Design review of the part shown in the three views and the two pictorial views. Dimensions are in mm from the part's minimum x, y and z. Coordinates: 2 decimals unless noted, no trailing zeros. Loops run counter-clockwise (first coordinate to the right, second up) from the corner with the lowest first, then second, coordinate; pieces in that order, holes last. Notation, with made-up numbers: M 42,-14.75 L 69,-14.75 A24 ccw 69,7.25 Z; hole C 75,-35 d5. An arc over 180 degrees is marked long. Answer as a JSON object with one key per item and string values. Group by question number.
Item 1: Wall thickness on L1, parallel to Y at x = 50, z = 1.3: over which ranges is the line inside the solid? List them lowest first. Write a range as from..to.
Item 2: Add section B-B (x = 10). State the section outline as (y, z) points, then the cut area to 3 significant figures.
Item 3: Insertion check: pin 1 (1 mm diameter, centred on x = 15, z = 2.5, fed in from -Y). The pin has a flat end and moves straight along its axis. Give the tip position at first contact, or say it passes through.
Item 4: Add section A-A (y = 10). State the section outline as (x, z) points.
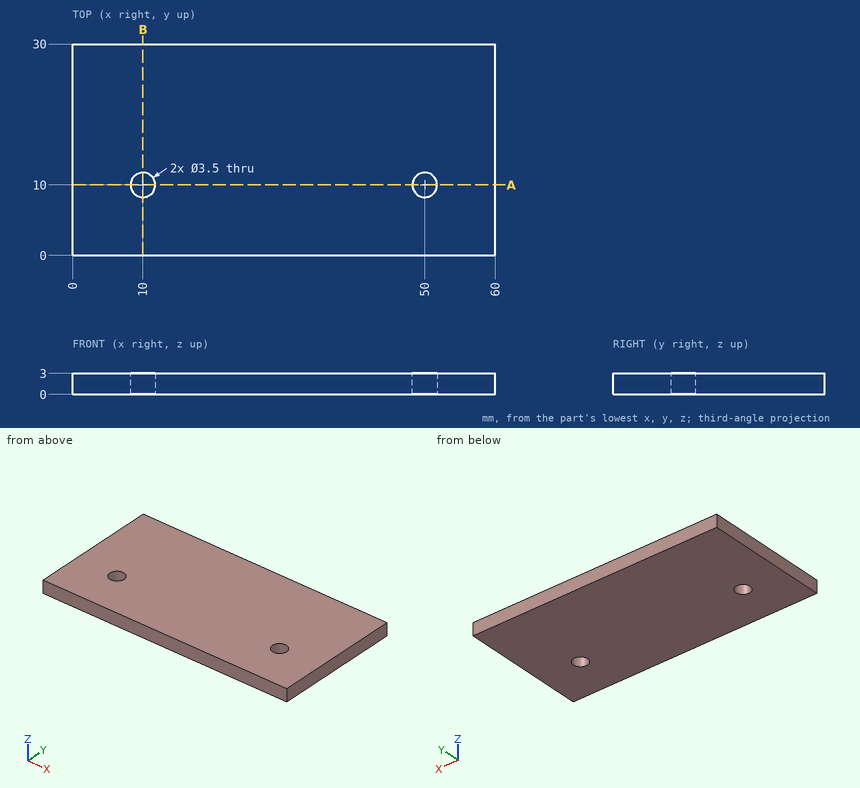
From the geometry:
{
 "1": {"L1": "y = 0..8.25, 11.75..30"},
 "2": {"outline": "M 0,0 L 8.25,0 L 8.25,3 L 0,3 Z; M 11.75,0 L 30,0 L 30,3 L 11.75,3 Z", "area": "79.5 mm²"},
 "3": {"pin 1": "stops at y = 0"},
 "4": {"outline": "M 0,0 L 8.25,0 L 8.25,3 L 0,3 Z; M 11.75,0 L 48.25,0 L 48.25,3 L 11.75,3 Z; M 51.75,0 L 60,0 L 60,3 L 51.75,3 Z"}
}
